Part print with two shaded views. Sizes in mm from the minimum x, y, z corner. A direction names the side the tool comes from. Round coordinates to 2 decimals unless told otherwise and drop trailing zeros. Order: outer loops, then holes, each group sorted by start corner. A loop starts at its lowest first (then second) coordinate and runs counter-clockwise, first axis right, second up. Notation, with made-up numbers: (-2.5, -18) -> (12.5, -18) arc R18 cw to (12.5, -9) -> close; hole circle Ø1 at (13, -26). An arc over 180 degrees is marked (long way). Answer as a JSON object with one key per item and string values.
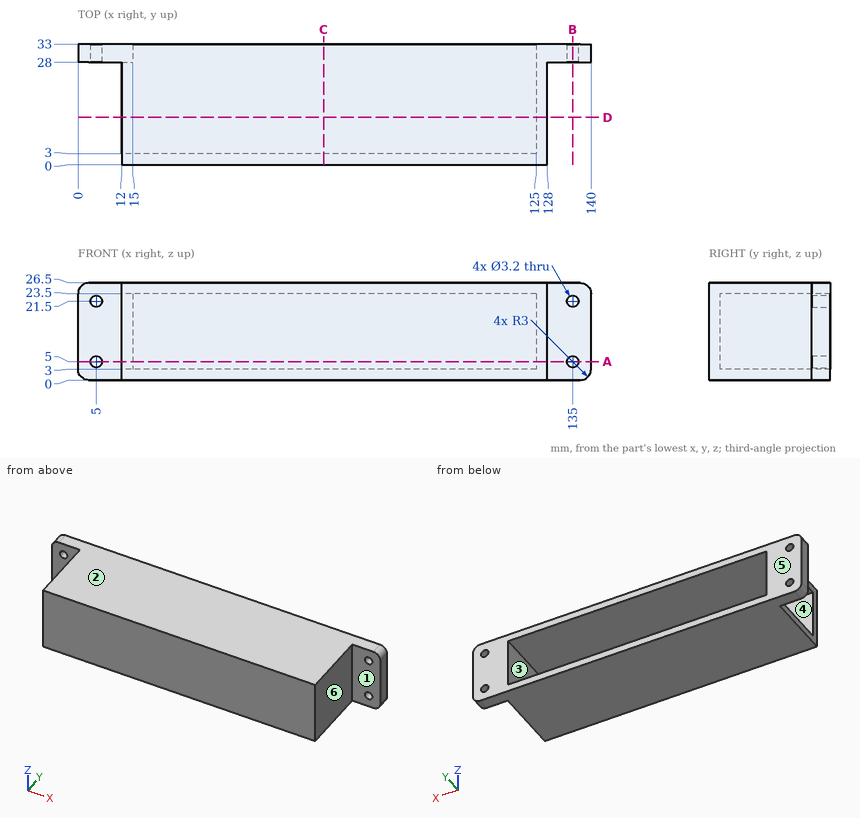
1) Cut at D-D, the plane y = 13. Give the cut face in (x, z).
Checked values:
{"outline": "(12, 0) -> (128, 0) -> (128, 26.5) -> (12, 26.5) -> (12, 23.5) -> (125, 23.5) -> (125, 3) -> (12, 3) -> close"}
2) Cut at B-B, the plane x = 135. Give the cut face in (y, z), plus the area to 4 significant figures.
Checked values:
{"outline": "(28, 0) -> (33, 0) -> (33, 3.4) -> (28, 3.4) -> close; (28, 6.6) -> (33, 6.6) -> (33, 19.9) -> (28, 19.9) -> close; (28, 23.1) -> (33, 23.1) -> (33, 26.5) -> (28, 26.5) -> close", "area": "100.5 mm²"}
3) Flat gauge pins, fed straight in: pin 1 Ø1.9 at (x, z) = (135, 21.5) entering from +Y; pin 2 Ø6 at (y, z) = (11.5, 9) entering from -X; pin 3 Ø13 at (y, z) = (12.5, 18) entering from -X; pin 4 Ø8 at (y, z) = (12.5, 10) entering from +X. Where does each tip first touch, or does it go through?
Checked values:
{"pin 1": "passes through", "pin 2": "stops at x = 125", "pin 3": "stops at x = 12", "pin 4": "stops at x = 128"}
4) Which spindle directions (+Z, -Z, +X, -X, +Y, -Y) get a long thin tool onto all of the face, cutting with end or side? Do the marked faces 5 and 6. Say none if no direction does.
Checked values:
{"face 5": "+Z, -Z, +X, -X, +Y", "face 6": "+Z, -Z, +X, -Y"}
5) Cut at A-A, the plane z = 5. Give the cut face in (x, y).
Checked values:
{"outline": "(0, 28) -> (3.4, 28) -> (3.4, 33) -> (0, 33) -> close; (6.6, 28) -> (15, 28) -> (15, 33) -> (6.6, 33) -> close; (12, 0) -> (128, 0) -> (128, 28) -> (133.4, 28) -> (133.4, 33) -> (125, 33) -> (125, 3) -> (12, 3) -> close; (136.6, 28) -> (140, 28) -> (140, 33) -> (136.6, 33) -> close"}
6) Pull direction Z, two halves, no side cores. Call the marked faces 1, 2, 3 and 4: pulls with the +Z half, pulls with the -Z half, needs draft (parallel to the pull), parting line crosses it, or undercut.
Checked values:
{"face 1": "needs draft", "face 2": "pulls with the +Z half", "face 3": "undercut", "face 4": "undercut"}
7) Cut at C-C, the plane x = 67. Give the cut face in (y, z).
Checked values:
{"outline": "(0, 0) -> (33, 0) -> (33, 3) -> (3, 3) -> (3, 23.5) -> (33, 23.5) -> (33, 26.5) -> (0, 26.5) -> close"}
8) Probe L1, parallel to Z at x = 135, y = 30; L2, parallel to Z at x = 53, y = 8; L3, parallel to Y at x = 91, z = 20.5. List the from-to ranges inside material, lowest first. Write a range as from..to.
Checked values:
{"L1": "z = 0..3.4, 6.6..19.9, 23.1..26.5", "L2": "z = 0..3, 23.5..26.5", "L3": "y = 0..3"}
